```python
from build123d import *

# Parameters (mm, degrees)
BOSS_EXTRUDE1_DEPTH   = 4
BOSS_EXTRUDE2_START   = -4
SKETCH2_W             = 12
SKETCH2_H             = 16
BOSS_EXTRUDE2_DEPTH   = 13
SKETCH3_W             = 12
SKETCH3_H             = 9
CUT_EXTRUDE1_DEPTH    = 9.5
SKETCH4_R             = 1
CUT_EXTRUDE2_DEPTH    = 16
BOSS_EXTRUDE3_START   = 2.5
BOSS_EXTRUDE3_DEPTH   = 5
BOSS_EXTRUDE3_2_DEPTH = 5
BOSS_EXTRUDE3_3_DEPTH = 5
BOSS_EXTRUDE3_4_DEPTH = 5
BOSS_EXTRUDE4_DEPTH   = 10
SKETCH6_R             = 1
CUT_EXTRUDE5_DEPTH    = 25
SKETCH7_R             = 1
CUT_EXTRUDE6_DEPTH    = 25
FILLET2_R             = 2.5


with BuildPart() as part:
    # Sketch1 → Boss-Extrude1 (new body)
    with BuildSketch(Plane.XY):
        Polygon((-30, 0), (30, 0), (0, 30), align=None)
    extrude(amount=BOSS_EXTRUDE1_DEPTH)

    # Sketch2 → Boss-Extrude2 (add)
    with BuildSketch(Plane.XY.offset(4).offset(BOSS_EXTRUDE2_START)):
        with Locations((0, -8)):
            Rectangle(SKETCH2_W, SKETCH2_H)
    extrude(amount=BOSS_EXTRUDE2_DEPTH)

    # Sketch3 → Cut-Extrude1 (cut)
    with BuildSketch(Plane.XY.offset(13)):
        with Locations((0, -8)):
            Rectangle(SKETCH3_W, SKETCH3_H)
    extrude(amount=-CUT_EXTRUDE1_DEPTH, mode=Mode.SUBTRACT)

    # Sketch4 → Cut-Extrude2 (cut)
    with BuildSketch(Plane.XZ.offset(16)):
        with Locations(Location((0, 9, 0), (0, 0, 270))):
            Circle(SKETCH4_R)
    extrude(amount=-CUT_EXTRUDE2_DEPTH, mode=Mode.SUBTRACT)



with BuildPart() as body_2:
    # Sketch5 → Boss-Extrude3 (new body)
    with BuildSketch(Plane.XY.offset(4).offset(BOSS_EXTRUDE3_START)):
        Polygon((-8.409009742, 15.934136008), (-14.065863992, 21.590990258), (-11.590990258, 24.065863992), (-5.934136008, 18.409009742), align=None)
    extrude(amount=BOSS_EXTRUDE3_DEPTH)


with BuildPart() as body_3:
    # Sketch5 → Boss-Extrude3 2 (new body)
    with BuildSketch(Plane.XY.offset(4).offset(BOSS_EXTRUDE3_START)):
        Polygon((-20.409009742, 3.934136008), (-26.065863992, 9.590990258), (-23.590990258, 12.065863992), (-17.934136008, 6.409009742), align=None)
    extrude(amount=BOSS_EXTRUDE3_2_DEPTH)


with BuildPart() as body_4:
    # Sketch5 → Boss-Extrude3 3 (new body)
    with BuildSketch(Plane.XY.offset(4).offset(BOSS_EXTRUDE3_START)):
        Polygon((8.621141777, 15.722003974), (14.277996026, 21.378858223), (16.75286976, 18.903984489), (11.096015511, 13.24713024), align=None)
    extrude(amount=BOSS_EXTRUDE3_3_DEPTH)


with BuildPart() as body_5:
    # Sketch5 → Boss-Extrude3 4 (new body)
    with BuildSketch(Plane.XY.offset(4).offset(BOSS_EXTRUDE3_START)):
        Polygon((20.621141777, 3.722003974), (26.277996026, 9.378858223), (28.75286976, 6.903984489), (23.096015511, 1.24713024), align=None)
    extrude(amount=BOSS_EXTRUDE3_4_DEPTH)


with BuildPart() as part_1:
    add(part.part)

    add(body_2.part)  # Boss-Extrude4 merges body 2

    add(body_3.part)  # Boss-Extrude4 merges body 3

    add(body_4.part)  # Boss-Extrude4 merges body 4

    add(body_5.part)  # Boss-Extrude4 merges body 5
    # Sketch8 → Boss-Extrude4 (add)
    with BuildSketch(Plane.XY.offset(11.5)):
        Polygon((-20.409009742, 3.934136008), (-17.934136008, 6.409009742), (-20.77228069, 9.247154424), (-23.247154424, 6.77228069), align=None)
        Polygon((-8.409009742, 15.934136008), (-5.934136008, 18.409009742), (-8.770090905, 21.24496464), (-11.24496464, 18.770090905), align=None)
        Polygon((8.621141777, 15.722003974), (11.096015511, 13.24713024), (13.908555635, 16.059670364), (11.433681901, 18.534544098), align=None)
        Polygon((23.096015511, 1.24713024), (20.621141777, 3.722003974), (23.433669477, 6.534531674), (25.908543211, 4.05965794), align=None)
    extrude(amount=-BOSS_EXTRUDE4_DEPTH)

    # Sketch6 → Cut-Extrude5 (cut)
    with BuildSketch(Plane(origin=(10.924442636, -10.924442636, 0), x_dir=(0.7071067811865506, 0.7071067811865446, 0), z_dir=(0.7071067811865446, -0.7071067811865506, 0))):
        with Locations((22.098203436, 9)):
            Circle(SKETCH6_R)
    extrude(amount=-CUT_EXTRUDE5_DEPTH, mode=Mode.SUBTRACT)

    # Sketch7 → Cut-Extrude6 (cut)
    with BuildSketch(Plane(origin=(-8.237436867, -8.237436867, 0), x_dir=(0, 0, 1), z_dir=(-0.7071067811865501, -0.7071067811865449, 0))):
        with Locations(Location((9, 22.098203436, 0), (0, 0, 270))):
            Circle(SKETCH7_R)
    extrude(amount=-CUT_EXTRUDE6_DEPTH, mode=Mode.SUBTRACT)

    # Fillet2
    fillet2_edges = [part_1.edges().sort_by_distance(p)[0] for p in [
        (15.515432893, 20.141421356, 11.5),
        (15.515432893, 20.141421356, 6.5),
        (27.515432893, 8.141421356, 6.5),
        (27.515432893, 8.141421356, 11.5),
        (-24.828427125, 10.828427125, 6.5),
        (-12.828427125, 22.828427125, 6.5),
        (-12.828427125, 22.828427125, 11.5),
        (-24.828427125, 10.828427125, 11.5),
    ]]
    fillet(fillet2_edges, radius=FILLET2_R - 0.0001)  # a hair under: the kernel refuses the full size


solid = part_1.part
```
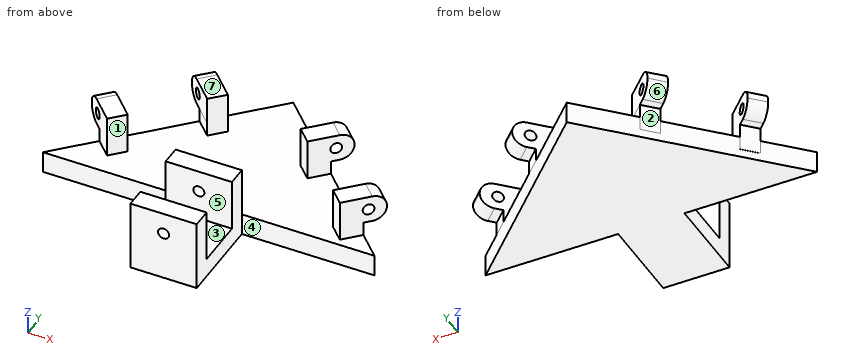
Could you check a few things on this model? Use its own coordinates, in mm. Face numbers are marked on the shaded views. A direction names the side the tool comes from. Round coordinates to 2 decimals unless told otherwise and drop trailing zeros. Loops run counter-clockwise (first coordinate to the right, second up) from the corner with the lowest first, then second, coordinate; pieces in that order, holes last. Notation, with made-up numbers: M 23,-8 L 42,-8 A9 cw 42,9 Z; hole C 51,-1 d7. An arc over 180 degrees is marked long. Answer as CSV lines item,"result".
1) We'd pull the mould along Y, two halves only. Please class the marked faces 5, 6 and 7: released by +Y, released by -Y, zero draft, split by the parting line, or undercut.
From the geometry:
face 5,"undercut"
face 6,"released by +Y"
face 7,"zero draft"
2) For pin 1 Ø15 at (x, y) = (-5.5, 15.5) entering from +Z; pin 2 Ø5 at (x, z) = (-11.5, 6) entering from +Y; pin 3 Ø1 at (x, y) = (-12.5, 24.5) entering from -Z; pin 4 Ø4.5 at (x, z) = (19, 2) entering from -Y, each with a flat end and sliding along its axis, tell me the tip position at first contact or that it passes through.
From the geometry:
pin 1,"z = 11.5"
pin 2,"y = 24.03"
pin 3,"through"
pin 4,"y = 0"
3) Imagine slicing it at A-A on y = -2. List the corners of the cut face in (x, z) for me.
From the geometry:
outline,"M -6,0 L 6,0 L 6,13 L -6,13 Z; hole C 0,9 d2"
4) If I drill on probe 1 along X at (y, z) = (-2.6, 9); probe 2 along Y at (x, z) = (4.5, 8.5); probe 3 along X at (y, z) = (24, 1), over which ranges is the centre line in solid material (lowest first)?
From the geometry:
probe 1,"-6 to -1, 1 to 6"
probe 2,"-16 to -12.5, -3.5 to 0"
probe 3,"-6 to 6"
5) Imagine slicing it at D-D on y = -10. List the corners of the cut face in (x, z) for me.
From the geometry:
outline,"M -6,0 L 6,0 L 6,3.5 L -6,3.5 Z"
6) Imagine slicing it at B-B on x = -3.5. List the corners of the cut face in (y, z) for me, and give its area (4 significant figures).
From the geometry:
outline,"M -16,0 L 26.5,0 L 26.5,4 L 0,4 L 0,13 L -3.5,13 L -3.5,3.5 L -12.5,3.5 L -12.5,13 L -16,13 Z"
area,"228.5 mm^2"
7) Which directions (+Z, -Z, +X, -X, +Y, -Y) give clear straight access to the entire face, cutting with the end or side of a thin tool? Please do the marked faces 1, 2, 3 and 4.
From the geometry:
face 1,"+Z, -Y"
face 2,"-Z, -X, +Y"
face 3,"+Z, +X, -X"
face 4,"+Z, -Z, +X, -Y"
